```python
from build123d import *

# Parameters (mm, degrees)
BOSS_EXTRUDE1_DEPTH = 38.1
SKETCH4_R           = 9.525
SKETCH4_R_2         = 6.35
CUT_EXTRUDE1_DEPTH  = 76.2


with BuildPart() as part:
    # Sketch3 → Boss-Extrude1 (new, symmetric)
    with BuildSketch(Plane.XY):
        with BuildLine():
            Line((-308.473797305, 97.683602722), (-254.535984299, 97.683602722))
            ThreePointArc((-254.535984299, 97.683602722), (-241.065600117, 92.103986904), (-235.485984299, 78.633602722))
            Line((-235.485984299, 78.633602722), (-235.485984299, 56.408602722))
            ThreePointArc((-235.485984299, 56.408602722), (-229.90636848, 42.938218541), (-216.435984299, 37.358602722))
            Line((-216.435984299, 37.358602722), (-159.285984299, 37.358602722))
            ThreePointArc((-159.285984299, 37.358602722), (-145.815600117, 42.938218541), (-140.235984299, 56.408602722))
            Line((-140.235984299, 56.408602722), (-140.235984299, 78.633602722))
            ThreePointArc((-140.235984299, 78.633602722), (-134.65636848, 92.103986904), (-121.185984299, 97.683602722))
            Line((-121.185984299, 97.683602722), (-67.173797305, 97.683602722))
            Line((-67.173797305, 97.683602722), (-67.173797305, 89.733402722))
            Line((-67.173797305, 89.733402722), (-121.185984299, 89.733402722))
            ThreePointArc((-121.185984299, 89.733402722), (-129.034728149, 86.482346572), (-132.285784299, 78.633602722))
            Line((-132.285784299, 78.633602722), (-132.285784299, 56.408602722))
            ThreePointArc((-132.285784299, 56.408602722), (-140.193959785, 37.316578209), (-159.285984299, 29.408402722))
            Line((-159.285984299, 29.408402722), (-216.435984299, 29.408402722))
            ThreePointArc((-216.435984299, 29.408402722), (-235.528008812, 37.316578209), (-243.436184299, 56.408602722))
            Line((-243.436184299, 56.408602722), (-243.436184299, 78.633602722))
            ThreePointArc((-243.436184299, 78.633602722), (-246.687240449, 86.482346572), (-254.535984299, 89.733402722))
            Line((-254.535984299, 89.733402722), (-308.473797305, 89.733402722))
            Line((-308.473797305, 89.733402722), (-308.473797305, 97.683602722))
        make_face()
    extrude(amount=BOSS_EXTRUDE1_DEPTH, both=True)

    # Sketch4 → Cut-Extrude1 (cut)
    with BuildSketch(Plane(origin=(0, 97.683602722, 0), x_dir=(1, 0, 0), z_dir=(0, 1, 0))):
        with Locations(Location((-190.5, 0, 0), (0, 0, 180))):
            Circle(SKETCH4_R)
        with Locations(Location((-285.859715502, 0, 0), (0, 0, 270))):
            Circle(SKETCH4_R_2)
        with Locations(Location((-92.710517543, 0, 0), (0, 0, 270))):
            Circle(SKETCH4_R_2)
    extrude(amount=-CUT_EXTRUDE1_DEPTH, mode=Mode.SUBTRACT)


solid = part.part
```
The model under review builds one solid part; all positions refer to its coordinate system, in mm. A direction names the side the tool comes from. Round coordinates to 2 decimals unless told otherwise and drop trailing zeros. Write each loop counter-clockwise with the first axis right and the second up, starting at its lowest first coordinate (ties: lowest second). Pieces come first, ordered by that corner, then holes. Notation, with made-up numbers: (-17.75, 20.5) - (-6.75, 20.5) arc R20 ccw to (-6.75, 33.5) - close; hole circle Ø5 at (53, 19.25). An arc over 180 degrees is marked (long way). Answer as CSV lines item,"result". Start each with the question number.
(1) To check wall thickness, follow line 1 (X direction, y = 68, z = -1); line 2 (X direction, y = 94.25, z = 0); line 3 (X direction, y = 91.5, z = 0). State the ranges of each line that lie inside material, in increasing order.
(2) We need section B-B on y = 72. State the section outline as (x, z) points, plus the area to 3 significant figures.
(3) We need section D-D on z = 15.5. State the section outline as (x, y) points.
(4) For pin 1 Ø17 at (x, z) = (-198.5, -18.5) entering from +Y; pin 2 Ø11 at (y, z) = (71.5, -2) entering from -X; pin 3 Ø24.5 at (y, z) = (69.5, -10) entering from +X, all flat-tipped, find the tip position at first contact; note any pin that passes through.
(5) For faces 1 (the flat face through (-235.486, 68, 1)), 2 (the flat face through (-187, 36, 38.1)), 3 (the flat face through (-132.286, 68, 1)), 4 (the flat face through (-243.436, 67, 1)), list the 3-axis set-ups (+Z, -Z, +X, -X, +Y, -Y) from which the entire face can be reached by the end or side of a thin tool; tool diameter is ignored.
(6) Draft analysis for pull direction X (two halves, no side actions). For faces 5 (the cylindrical face through (-292.059, 93.764, -1.377)), 6 (the cylindrical face through (-134.8, 91.96, 0.53)), 7 (the cylindrical face through (-139.985, 37.528, 0.533)), 8 (the flat face through (-308.474, 94, 1)), state which applies: pulls with the +X half, pulls with the -X half, needs draft (parallel to the pull), parting line crosses it, or undercut.
(7) We need section C-C on z = 0. Give the number of separate pieces and of enclosed holes in the cut face, plus the area to 3 significant figures.
(8) We need section A-A on x = -190.5. State the section outline as (y, z) points (3 decimals), plus the area to 3 significant figures.
Worked answers:
1,line 1,"-243.44 to -235.49, -140.24 to -132.29"
1,line 2,"-308.47 to -292.21, -279.51 to -243.63, -132.1 to -99.06, -86.36 to -67.17"
1,line 3,"-308.47 to -292.21, -279.51 to -240.49, -135.23 to -99.06, -86.36 to -67.17"
2,outline,"(-243.44, -38.1) - (-235.49, -38.1) - (-235.49, 38.1) - (-243.44, 38.1) - close; (-140.24, -38.1) - (-132.29, -38.1) - (-132.29, 38.1) - (-140.24, 38.1) - close"
2,area,"1,210 mm²"
3,outline,"(-308.47, 89.73) - (-254.54, 89.73) arc R11.1 cw to (-243.44, 78.63) - (-243.44, 56.41) arc R27 ccw to (-216.44, 29.41) - (-159.29, 29.41) arc R27 ccw to (-132.29, 56.41) - (-132.29, 78.63) arc R11.1 cw to (-121.19, 89.73) - (-67.17, 89.73) - (-67.17, 97.68) - (-121.19, 97.68) arc R19.05 ccw to (-140.24, 78.63) - (-140.24, 56.41) arc R19.05 cw to (-159.29, 37.36) - (-216.44, 37.36) arc R19.05 cw to (-235.49, 56.41) - (-235.49, 78.63) arc R19.05 ccw to (-254.54, 97.68) - (-308.47, 97.68) - close"
4,pin 1,"y = 37.36"
4,pin 2,"x = -243.44"
4,pin 3,"x = -131.84"
5,face 1,"+Z, -Z, +Y"
5,face 2,"+Z, +X, -X, +Y, -Y"
5,face 3,"+Z, -Z, +X, -Y"
5,face 4,"+Z, -Z, -X, -Y"
6,face 5,"undercut"
6,face 6,"undercut"
6,face 7,"pulls with the +X half"
6,face 8,"pulls with the -X half"
7,separate pieces,"4"
7,enclosed holes,"0"
7,area,"2,260 mm²"
8,outline,"(29.408, -38.1) - (37.359, -38.1) - (37.359, -9.525) - (29.408, -9.525) - close; (29.408, 9.525) - (37.359, 9.525) - (37.359, 38.1) - (29.408, 38.1) - close"
8,area,"454 mm²"
